Geometry check sheet. Reference: the model listing, model coordinates, mm. A direction names the side the tool comes from. Round coordinates to 2 decimals unless told otherwise and drop trailing zeros. Loops run counter-clockwise (first coordinate to the right, second up) from the corner with the lowest first, then second, coordinate; pieces in that order, holes last.
```python
from build123d import *

# Parameters (mm, degrees)
SKETCH4_R           = 1.25
BOSS_EXTRUDE1_DEPTH = 5
CUT_EXTRUDE1_DEPTH  = 10


with BuildPart() as part:
    # Sketch4 → Boss-Extrude1 (new body)
    with BuildSketch(Plane(origin=(0, 0, 0), x_dir=(1, 0, 0), z_dir=(0, 1, 0))):
        Polygon((79, -2.5), (79, -5), (79, -7.5), (79, -8.25), (82.9, -8.25), (82.9, -10.15), (89, -10.15), (89, -2.5), align=None)
        with Locations((81.5, -5)):
            Circle(SKETCH4_R, mode=Mode.SUBTRACT)
    extrude(amount=BOSS_EXTRUDE1_DEPTH)

    # Sketch5 → Cut-Extrude1 (cut)
    with BuildSketch(Plane(origin=(89, 0, 0), x_dir=(0, 0, -1), z_dir=(1, 0, 0))):
        with BuildLine():
            ThreePointArc((-5, 2.5), (-5.366116524, 3.383883476), (-6.25, 3.75))
            Line((-6.25, 3.75), (-6.25, 1.25))
            ThreePointArc((-6.25, 1.25), (-5.366116524, 1.616116524), (-5, 2.5))
        make_face()
        with BuildLine():
            Line((-6.25, 1.25), (-6.25, 3.75))
            ThreePointArc((-6.25, 3.75), (-7.5, 2.5), (-6.25, 1.25))
        make_face()
    extrude(amount=-CUT_EXTRUDE1_DEPTH, mode=Mode.SUBTRACT)


solid = part.part
```
1) Sectioned sample at B-B, the plane y = 2.7. Record the cut outline in (x, z).
Report:
outline: (79, 2.5) - (89, 2.5) - (89, 5.02) - (82.75, 5.02) arc R1.25 cw (long way) to (80.25, 5.02) - (79, 5.02) - close; (79, 7.48) - (89, 7.48) - (89, 10.15) - (82.9, 10.15) - (82.9, 8.25) - (79, 8.25) - close
2) Sectioned sample at C-C, the plane y = 0.45. Record the cut outline in (x, z).
Report:
outline: (79, 2.5) - (89, 2.5) - (89, 10.15) - (82.9, 10.15) - (82.9, 8.25) - (79, 8.25) - close; hole circle Ø2.5 at (81.5, 5)
3) Sectioned sample at A-A, the plane x = 83.75. Record the cut outline in (y, z).
Report:
outline: (0, 2.5) - (5, 2.5) - (5, 10.15) - (0, 10.15) - close; hole circle Ø2.5 at (2.5, 6.25)
4) Scan lines: line 1 along X through (y, z) = (1.4, 5); line 2 along Z through (x, y) = (81.5, 3.1); line 3 along Z through (x, y) = (82, 2.25). Record each from-to range of solid material in increasing order.
Report:
line 1: x = 79 to 80.25, 82.75 to 89
line 2: z = 2.5 to 3.75, 7.35 to 8.25
line 3: z = 2.5 to 3.85, 7.47 to 8.25
5) Sectioned sample at D-D, the plane x = 82. Record the cut outline in (y, z).
Report:
outline: (0, 2.5) - (5, 2.5) - (5, 3.85) - (0, 3.85) - close; (0, 6.15) - (1.25, 6.15) arc R1.25 cw (long way) to (3.75, 6.15) - (5, 6.15) - (5, 8.25) - (0, 8.25) - close
6) Access from +Z, -Z, +X, -X, +Y, -Y to the whole of each face (thin tool, end or side, straight path). Record for faces 1 (the face through (86, 2, 10.15)), 2 (the face through (81, 2, 8.25)).
Report:
face 1: +Z, +X, -X, +Y, -Y
face 2: +Z, -X, +Y, -Y
7) Mould release check, pull along X, two halves, no side actions. Record for faces 3 (the face through (89, 1, 6)), 4 (the face through (82.9, 2, 9)), 5 (the face through (84, 2, 2.5)), 6 (the face through (81.34, 2.46, 3.76)): +X half, -X half, draft (parallel to the pull), parting line (faces both ways), or undercut.
Report:
face 3: +X half
face 4: -X half
face 5: draft
face 6: undercut
8) Gauge pin test, flat end, axial feed: pin 1 (1.2 mm diameter, centred on x = 80.5, y = 3.5, fed in from +Z). Record the tip position at first contact, or that the pin passes through.
Report:
pin 1: stops at z = 8.25
